Build history of the part. All positions in model axes, mm. Round coordinates to 2 decimals unless told otherwise and drop trailing zeros. Loops run counter-clockwise (first coordinate to the right, second up) from the corner with the lowest first, then second, coordinate; pieces in that order, holes last. Notation, with made-up numbers: M 83,46 L 137,46 A24 cw 137,76 Z; hole C 74.25,80.5 d8. An arc over 180 degrees is marked long. Write each question's results on one line, items separated by ' | '. Start each with the question number.
```python
from build123d import *

# Parameters (mm, degrees)
SKIZZE1_R                       = 21.035
SKIZZE1_R_2                     = 17.525
AUFSATZ_LINEAR_AUSTRAGEN1_DEPTH = 375
SKIZZE2_W                       = 50
SKIZZE2_H                       = 630
SCHNITT_LINEAR_AUSTRAGEN1_DEPTH = 377.178072793


with BuildPart() as part:
    # Skizze1 → Aufsatz-Linear austragen1 (new, symmetric)
    with BuildSketch(Plane.XY):
        Circle(SKIZZE1_R)
        Circle(SKIZZE1_R_2, mode=Mode.SUBTRACT)
    extrude(amount=AUFSATZ_LINEAR_AUSTRAGEN1_DEPTH, both=True)

    # Skizze2 → Schnitt-Linear austragen1 (cut, through all)
    with BuildSketch(Plane(origin=(0, 0, 0), x_dir=(1, 0, 0), z_dir=(0, 1, 0))):
        with Locations((25, 0)):
            Rectangle(SKIZZE2_W, SKIZZE2_H)
    extrude(amount=SCHNITT_LINEAR_AUSTRAGEN1_DEPTH, mode=Mode.SUBTRACT)


solid = part.part
```
Item 1: Saw through at B-B, the plane z = 21. Give the cut face in (x, y) (3 decimals).
Item 2: Mould opens along Z. For faces 1 (the flat face through (-8, 16, -375)), 2 (the flat face through (13, 13, -315)), 3 (the flat face through (13, 13, 315)), 4 (the cylindrical face through (-13.91, -10.66, -5.25)) say: released by +Z, released by -Z, zero draft, split by the parting line, or undercut.
Item 3: Saw through at A-A, the plane z = 323. Give the cut face in (x, y) (3 decimals).
Item 4: Drop flat-ended pins along their axis: pin 1 (5 mm diameter, centred on y = -4.5, z = 26, fed in from -X); pin 2 (3 mm diameter, centred on y = 5.5, z = -262.5, fed in from +X); pin 3 (12 mm diameter, centred on x = -16, z = -173.5, fed in from -Y); pin 4 (6 mm diameter, centred on x = -10, y = 10, fed in from +Z). Give the stop position or say it passes through.
Item 5: Drill centre lines: line 1 along Z through (x, y) = (17, 10); line 2 along X through (y, z) = (-1.5, 84); line 3 along Y through (x, z) = (-9, -195). Where is each one in solid material? Low to high. Write a range as [from, to].
Working result:
1) outline: M 0,17.525 L 0,21.035 A21.035 ccw long 21.035,0 L 17.525,0 A17.525 cw long Z
2) face 1: released by -Z | face 2: undercut | face 3: undercut | face 4: zero draft
3) outline: C 0,0 d42.07; hole C 0,0 d35.05
4) pin 1: stops at x = -20.94 | pin 2: stops at x = -16.07 | pin 3: stops at y = -18.51 | pin 4: passes through
5) line 1: z = [-375, -315], [315, 375] | line 2: x = [-20.98, -17.46], [17.46, 20.98] | line 3: y = [-19.01, -15.04], [15.04, 19.01]
